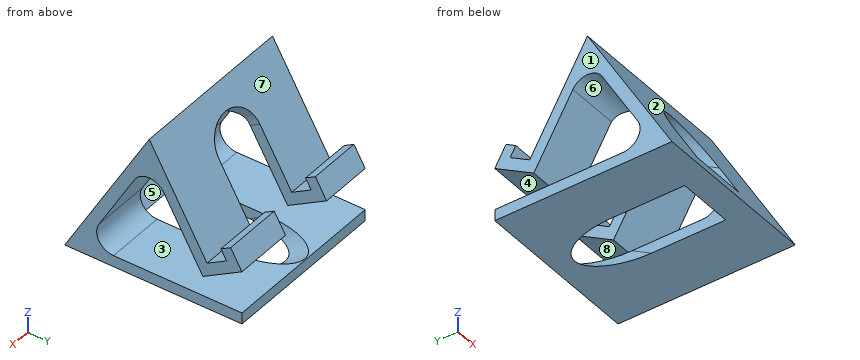
from build123d import *

# Parameters (mm, degrees)
PAD_DEPTH    = 75
POCKET_DEPTH = 70


with BuildPart() as part:
    # Sketch → Pad (new body)
    with BuildSketch(Plane.YZ):
        with BuildLine():
            Line((0, 0), (37.5, 64.951905))
            Line((37.5, 64.951905), (63.169873, 20.490381))
            Line((71.830127, 25.490381), (63.169873, 20.490381))
            Line((69.330127, 29.820508), (71.830127, 25.490381))
            Line((73.660254, 32.320508), (69.330127, 29.820508))
            Line((78.660254, 23.660254), (73.660254, 32.320508))
            Line((61.339746, 13.660254), (78.660254, 23.660254))
            Line((43.995191, 43.701905), (61.339746, 13.660254))
            ThreePointArc((43.995191, 43.701905), (37.5, 47.451905), (31.004809, 43.701905))
            Line((15.155445, 16.25), (31.004809, 43.701905))
            ThreePointArc((15.155445, 16.25), (15.155445, 8.75), (21.650635, 5))
            Line((21.650635, 5), (66.339746, 5))
            Line((66.339746, 5), (78.660254, 5))
            Line((78.660254, 5), (78.660254, 0))
            Line((0, 0), (78.660254, 0))
        make_face()
    extrude(amount=PAD_DEPTH)

    # Sketch001 (on DatumPlane) → Pocket (cut)
    with BuildSketch(Plane(origin=(0, 69.240381, 39.975953), x_dir=(0, -0.5, 0.866025), z_dir=(0, 0.866025, 0.5))):
        with BuildLine():
            ThreePointArc((14.354353, 23.5), (26.854353, 36), (14.354353, 48.5))
            Line((14.354353, 48.5), (-22.231963, 48.5))
            ThreePointArc((-22.231963, 48.5), (-34.731963, 36), (-22.231963, 23.5))
            Line((-22.231963, 23.5), (14.354353, 23.5))
        make_face()
    extrude(amount=-POCKET_DEPTH, mode=Mode.SUBTRACT)


solid = part.part
Can you work these out from the model? Positions are in its coordinate system, mm. Face numbers are marked on the shaded views. A direction names the side the tool comes from. Coordinates: 2 decimals unless noted, no trailing zeros. Loops run counter-clockwise (first coordinate to the right, second up) from the corner with the lowest first, then second, coordinate; pieces in that order, holes last. Notation, with made-up numbers: (71.5, -15.5) - (117.5, -15.5) arc R13 cw to (117.5, -8.5) - close; hole circle Ø9 at (9.25, 0). An arc over 180 degrees is marked (long way). Answer as a JSON object with one key per item and string values. Group by question number.
Item 1: If we mould it in two halves opening along Z, with no side actions, what happens to the marked faces 1, 2, 3 and 4? For each: released by +Z, released by -Z, zero draft, split by the parting line, or undercut.
Item 2: If I drill on L1, parallel to Y at x = 58, z = 21.5; L2, parallel to Y at x = 17, z = 32; L3, parallel to X at y = 13.5, z = 21, over which ranges is the centre line in solid material (lowest first)? Write a range as from..to.
Item 3: If we section it at C-C (x = 58): List the corners of the cut face in (y, z) for me.
Item 4: On a 3-axis mill with a long thin cutter (end or side, diameter ignored), from which of +Z, -Z, +X, -X, +Y, -Y can I reach the whole of each face in a straight line? I mean the marked faces 5, 6, 7 and 8. Say none if no direction works.
Item 5: If we section it at B-B (y = 9): List the corners of the cut face in (x, z) for me.
Item 6: If we section it at D-D (z = 46): State how many separate pieces and enclosed holes the cut face has, plus the area to 3 significant figures.
Item 7: If we section it at A-A (x = 40.5): List the corners of the cut face in (y, z) for me, plus the area to 3 significant figures.
Item 8: For pin 1 (10 mm diameter, centred on x = 50.5, z = 12.5, fed in from -Y); pin 2 (1 mm diameter, centred on x = 18.5, z = 18.5, fed in from -Y); pin 3 (4 mm diameter, centred on x = 60, z = 39.5, fed in from +Y), each with a flat end and sliding along its axis, tell me the tip position at first contact or that it passes through.
Returned:
{
 "1": {"face 1": "zero draft", "face 2": "released by +Z", "face 3": "undercut", "face 4": "undercut"},
 "2": {"L1": "y = 12.41..18.19, 56.81..62.59, 64.92..74.92", "L2": "y = 18.48..24.25, 50.75..56.52, 73.11..73.85", "L3": "x = 0..23.5, 48.5..75"},
 "3": {"outline": "(0, 0) - (78.66, 0) - (78.66, 5) - (21.65, 5) arc R7.5 cw to (15.16, 16.25) - (31, 43.7) arc R7.5 cw to (44, 43.7) - (61.34, 13.66) - (78.66, 23.66) - (73.66, 32.32) - (69.33, 29.82) - (71.83, 25.49) - (63.17, 20.49) - (37.5, 64.95) - close"},
 "4": {"face 5": "+Z", "face 6": "+X, -X", "face 7": "+Z, +X, -X", "face 8": "+X, -X, +Y"},
 "5": {"outline": "(0, 0) - (75, 0) - (75, 15.59) - (48.5, 15.59) - (48.5, 4.32) - (23.5, 4.32) - (23.5, 15.59) - (0, 15.59) - close"},
 "6": {"separate pieces": "4", "enclosed holes": "0", "area": "735 mm²"},
 "7": {"outline": "(0, 0) - (11.49, 0) - (5.75, 9.95) - close; (26.02, 45.06) - (43.24, 55.01) - (37.5, 64.95) - close; (67.79, 0) - (78.66, 0) - (78.66, 5) - (76.45, 5) - close", "area": "204 mm²"},
 "8": {"pin 1": "stops at y = 4.33", "pin 2": "stops at y = 10.39", "pin 3": "stops at y = 53.35"}
}
